```python
from build123d import *

# Parameters (mm, degrees)
SKETCH2_W        = 44.45
SKETCH2_H        = 5.826125
SKETCH3_W        = 5.826125
SKETCH3_H        = 44.45
SWEEP1_OUTLINE_R = 31.0515
SWEEP1_ANGLE     = 90


# Read off the part's stored shape, not the designer's step: Sweep1
with BuildPart() as part:
    # Sketch2 → Revolve1 (revolve)
    with BuildSketch(Plane(origin=(0, 0, 0), x_dir=(0, 0, -1), z_dir=(1, 0, 0))):
        with Locations((-60.325, 39.5525625)):
            Rectangle(SKETCH2_W, SKETCH2_H)
    revolve(axis=Axis((0, 0, 0), (0, 0, 1)))

    # Sketch3 → Revolve2 (revolve)
    with BuildSketch(Plane(origin=(0, 0, 0), x_dir=(0, 0, -1), z_dir=(1, 0, 0))):
        with Locations((39.5525625, 60.325)):
            Rectangle(SKETCH3_W, SKETCH3_H)
    revolve(axis=Axis((0, 0, 0), (0, 1, 0)))

    # Sweep1 outline → Sweep1 (revolve)
    with BuildSketch(Plane(origin=(0, 38.1, 38.1), x_dir=(0, -1, 0), z_dir=(0, 0, 1))):
        with BuildLine():
            Line((0, 18.754181044), (0, -18.754181044))
            add(Edge.make_bspline(
                [(0, -18.754181044), (3.595121657, -26.057839615), (9.397449748, -33.407976072), (17.825883125, -39.559399853), (28.204619336, -42.465624968), (44.310790561, -42.46562502), (50.403307493, -41.329592494), (55.932569526, -39.150372881), (60.686650624, -36.321869277), (69.83985958, -28.979313764), (74.693549795, -23.427727825), (78.605101985, -16.344282836), (82.51560631, -3.11e-07), (78.605102252, 16.34428235), (74.693550018, 23.42772757), (69.839859698, 28.979313669), (60.686650629, 36.321869273), (55.932569539, 39.150372874), (50.403307515, 41.329592485), (44.310790594, 42.465625014), (28.204619371, 42.465624978), (17.825883146, 39.559399869), (9.397449758, 33.407976085), (3.59512166, 26.057839621), (0, 18.754181044)],
                knots=[3.599009571, 3.599009571, 3.599009571, 3.599009571, 3.599009571, 3.599009571, 4.698420057, 4.698420057, 4.698420057, 4.698420057, 5.388460062, 5.388460062, 5.388460062, 5.388460062, 6.283185297, 6.283185297, 6.283185297, 7.177910553, 7.177910553, 7.177910553, 7.177910553, 7.867950556, 7.867950556, 7.867950556, 7.867950556, 8.967361044, 8.967361044, 8.967361044, 8.967361044, 8.967361044, 8.967361044], degree=5, weights=[1, 1, 0.995343828, 0.991763785, 1, 1, 0.999483219, 0.999983206, 1, 1, 0.998916664, 0.997304294, 1.002695707, 0.997304293, 0.998916664, 1, 1, 0.999983206, 0.999483219, 1, 1, 0.991763785, 0.995343828, 1, 1]))
        make_face()
        with Locations((38.1, 0)):
            Circle(SWEEP1_OUTLINE_R, mode=Mode.SUBTRACT)
    revolve(axis=Axis((0, 38.1, 38.1), (1, 0, 0)), revolution_arc=SWEEP1_ANGLE)


solid = part.part
```
The listing builds one solid part. Answer for the finished solid, in the listing's coordinates (mm). A direction names the side the tool comes from. Coordinates: 2 decimals unless noted, no trailing zeros. Write each loop counter-clockwise with the first axis right and the second up, starting at its lowest first coordinate (ties: lowest second). Pieces come first, ordered by that corner, then holes.
Q1. Given P1, Ø5, axis at x = 23.5, z = -17, coming from the -Y side; P2, Ø1.5, axis at y = -16.5, z = 26, coming from the +X side; P3, Ø2, axis at x = 2, z = 66, coming from the +Y side, each flat-ended and moving along its own axis, determine where each tip first touches the part or whether it passes through.
Returned:
P1: stops at y = -14.05
P2: stops at x = 38.88
P3: stops at y = 42.45
Q2. Find the intervals of material crossed by line 1 along Z through (x, y) = (0, 51.5); line 2 along Y through (x, z) = (25.5, 40.5), in increasing order.
Returned:
line 1: z = -42.47 to -36.64, 36.64 to 42.47
line 2: y = -33.96 to -26.31, 26.31 to 33.96
Q3. Which of the six approach directions +Z, -Z, +X, -X, +Y, -Y give full straight-line access (tool end or side, diameter ignored) to faces 4 (the flat face through (19, 82.55, -32)), 5 (the flat face through (16, 38.1, 27)), 6 (the cylindrical face through (-11.006, 34.948, 60.014))?
Returned:
face 4: +Z, -Z, +X, -X, +Y
face 5: +Y
face 6: +Z
Q4. Section A-A, the plane z = 63 is taken. Write down the section's boundary in (x, y).
Returned:
outline: circle Ø84.93 at (0, 0); hole circle Ø73.28 at (0, 0)
Q5. The mould has two halves that part along X. Classify faces 1 (the flat face through (16, 27, 38.1)), 2 (the cylindrical face through (16.26, 60.64, -39.23)), 3 (the flat face through (19, 32, 82.55)): released by +X, released by -X, zero draft, split by the parting line, or undercut.
Returned:
face 1: undercut
face 2: split by the parting line
face 3: zero draft
